The listing builds one solid part. Answer for the finished solid, in the listing's coordinates (mm). Face numbers are marked on the shaded views. Round coordinates to 2 decimals unless told otherwise and drop trailing zeros. Order: outer loops, then holes, each group sorted by start corner. A loop starts at its lowest first (then second) coordinate and runs counter-clockwise, first axis right, second up. Notation, with made-up numbers: (-36.5, -22.5) -> (-12.5, -22.5) arc R31 cw to (-12.5, 2.5) -> close; hole circle Ø2 at (-34, 62.25). An arc over 180 degrees is marked (long way). Return JSON: item names as keys, results as strings. Group by question number.
(1) The part is cut by section D-D (z = 9). Determine the outline of the cut face in (x, y), plus the area to 3 significant figures.
(2) Consider line 1 (X direction, y = -6, z = 7.75); line 2 (Y direction, x = 12, z = -1.75); line 3 (Z direction, x = 0, y = -16.5). Determine where each line is inside the solid, lowest interval first. Write a range as [from, to].
(3) The part is cut by section B-B (z = 0). Determine the outline of the cut face in (x, y).
(4) The part is cut by section C-C (x = -12). Determine the outline of the cut face in (y, z).
(5) Determine the mould class of the marked faces 1, 2 and 3 for opening direction Z: +Z half, -Z half, draft (parallel to the pull), parting line (faces both ways), or undercut.
(6) The part is cut by section A-A (y = -6). Determine the outline of the cut face in (x, z).
from build123d import *

# Parameters (mm, degrees)
SKETCH_W     = 33.5
SKETCH_H     = 21.5
SKETCH_R     = 4
PAD_DEPTH    = 30
SKETCH001_R  = 1.7
POCKET_DEPTH = 21.501


with BuildPart() as part:
    # Sketch → Pad (new body)
    with BuildSketch(Plane.XZ):
        Rectangle(SKETCH_W, SKETCH_H)
        Circle(SKETCH_R, mode=Mode.SUBTRACT)
    extrude(amount=PAD_DEPTH)

    # Sketch001 → Pocket (cut, through all)
    with BuildSketch(Plane(origin=(0, 0, -10.75), x_dir=(1, 0, 0), z_dir=(0, 0, -1))):
        with Locations((-12, 24)):
            Circle(SKETCH001_R)
        with Locations((12, 24)):
            Circle(SKETCH001_R)
        with Locations((12, 6)):
            Circle(SKETCH001_R)
        with Locations((-12, 6)):
            Circle(SKETCH001_R)
    extrude(amount=-POCKET_DEPTH, mode=Mode.SUBTRACT)


solid = part.part
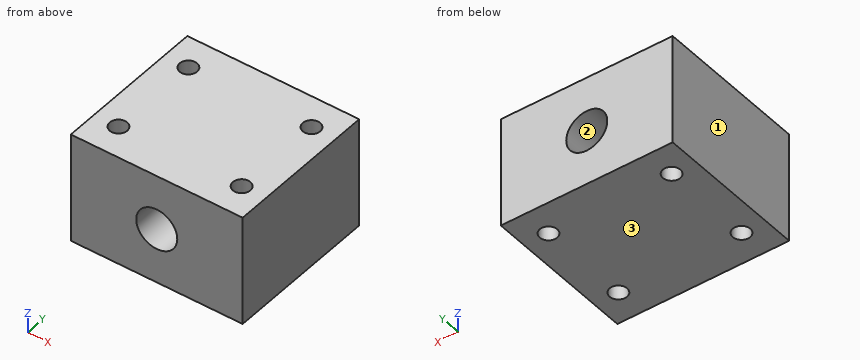
Answer below:
{
 "1": {"outline": "(-16.75, -30) -> (16.75, -30) -> (16.75, 0) -> (-16.75, 0) -> close; hole circle Ø3.4 at (-12, -24); hole circle Ø3.4 at (-12, -6); hole circle Ø3.4 at (12, -24); hole circle Ø3.4 at (12, -6)", "area": "969 mm²"},
 "2": {"line 1": "x = [-16.75, -13.7], [-10.3, 10.3], [13.7, 16.75]", "line 2": "y = [-30, -25.7], [-22.3, -7.7], [-4.3, 0]", "line 3": "z = [-10.75, -4], [4, 10.75]"},
 "3": {"outline": "(-16.75, -30) -> (-4, -30) -> (-4, 0) -> (-16.75, 0) -> close; (4, -30) -> (16.75, -30) -> (16.75, 0) -> (4, 0) -> close; hole circle Ø3.4 at (-12, -24); hole circle Ø3.4 at (-12, -6); hole circle Ø3.4 at (12, -24); hole circle Ø3.4 at (12, -6)"},
 "4": {"outline": "(-30, -10.75) -> (-25.7, -10.75) -> (-25.7, 10.75) -> (-30, 10.75) -> close; (-22.3, -10.75) -> (-7.7, -10.75) -> (-7.7, 10.75) -> (-22.3, 10.75) -> close; (-4.3, -10.75) -> (0, -10.75) -> (0, 10.75) -> (-4.3, 10.75) -> close"},
 "5": {"face 1": "draft", "face 2": "undercut", "face 3": "-Z half"},
 "6": {"outline": "(-16.75, -10.75) -> (-13.7, -10.75) -> (-13.7, 10.75) -> (-16.75, 10.75) -> close; (-10.3, -10.75) -> (10.3, -10.75) -> (10.3, 10.75) -> (-10.3, 10.75) -> close; (13.7, -10.75) -> (16.75, -10.75) -> (16.75, 10.75) -> (13.7, 10.75) -> close; hole circle Ø8 at (0, 0)"}
}
